Here's how the part is built. I have some questions about the finished solid (model axes, mm). Face numbers are marked on the shaded views. Coordinates: 2 decimals unless noted, no trailing zeros. Order: outer loops, then holes, each group sorted by start corner. A loop starts at its lowest first (then second) coordinate and runs counter-clockwise, first axis right, second up. Notation, with made-up numbers: (6, 24) - (63, 24) arc R28 cw to (63, 42) - close; hole circle Ø10 at (46.5, 20). An arc over 180 degrees is marked (long way). Use one line per item in the form item = value. Start each with the question number.
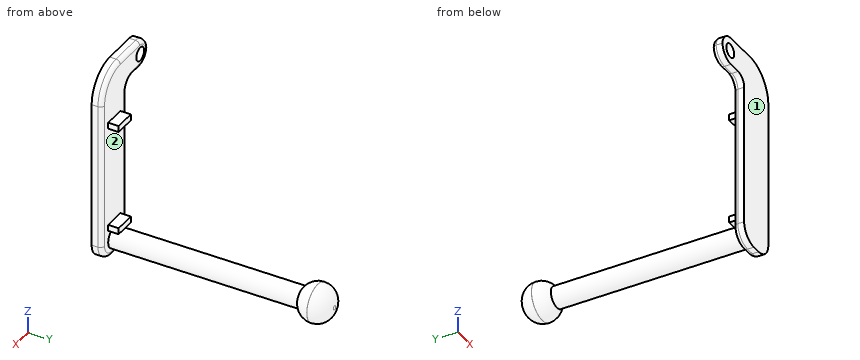
from build123d import *

# Parameters (mm, degrees)
SKETCH2_W           = 13
SKETCH2_H           = 13
SKETCH2_R           = 3.25
BOSS_EXTRUDE2_DEPTH = 5
FILLET1_R           = 15
FILLET2_R           = 5
FILLET3_R           = 7
FILLET4_R           = 2
FILLET5_R           = 8
SKETCH4_R           = 5
BOSS_EXTRUDE4_DEPTH = 90
SKETCH5_R           = 9
BOSS_EXTRUDE5_DEPTH = 15
FILLET6_R           = 8
SKETCH6_W           = 10
SKETCH6_H           = 1.5
BOSS_EXTRUDE6_DEPTH = 5
SKETCH7_W           = 10
SKETCH7_H           = 3
BOSS_EXTRUDE7_DEPTH = 5


with BuildPart() as part:
    # Sketch2 → Boss-Extrude2 (new body)
    # profile 1 of 2: a face of its own
    with BuildSketch(Plane(origin=(0, 0, 0), x_dir=(1, 0, 0), z_dir=(0, 1, 0))):
        with Locations((6.5, 6.5)):
            Rectangle(SKETCH2_W, SKETCH2_H)
        with Locations(Location((6.5, 6.5, 0), (0, 0, 270))):
            Circle(SKETCH2_R, mode=Mode.SUBTRACT)
    # profile 2 of 2: a face of its own
    with BuildSketch(Plane(origin=(0, 0, 0), x_dir=(1, 0, 0), z_dir=(0, 1, 0))):
        Polygon((13, 13), (13, 0), (38, 0), (38, 93), (18, 93), (18, 13), align=None)
    extrude(amount=BOSS_EXTRUDE2_DEPTH)

    # Fillet1
    fillet1_edges = [part.edges().sort_by_distance(p)[0] for p in [
        (38, 2.5, 0),
    ]]
    fillet(fillet1_edges, radius=FILLET1_R)

    # Fillet2
    fillet2_edges = [part.edges().sort_by_distance(p)[0] for p in [
        (18, 2.5, -13),
    ]]
    fillet(fillet2_edges, radius=FILLET2_R)

    # Fillet3
    # the kernel refuses this fillet: 7 mm, written as the material it takes off along each edge
    with BuildSketch(Plane(origin=(0, -17.5, 0), x_dir=(0, 0, -1), z_dir=(0, 1, 0)), Plane(origin=(0, -17.5, -13), x_dir=(1, 0, 0), z_dir=(0, 1, 0))) as fillet3_piece_1:
        with BuildLine():
            CenterArc((FILLET3_R, -FILLET3_R), FILLET3_R, 90, 90)
            Line((0, -FILLET3_R), (0, 0))
            Line((0, 0), (FILLET3_R, 0))
        make_face()
    extrude(amount=40, mode=Mode.SUBTRACT)

    # Fillet4
    # the kernel refuses this fillet: 2 mm, written as the material it takes off along each edge
    with BuildSketch(Plane(origin=(43, 5, -93), x_dir=(0, 0, 1), z_dir=(-1, 0, 0))) as fillet4_piece_1:
        with BuildLine():
            CenterArc((FILLET4_R, -FILLET4_R), FILLET4_R, 90, 90)
            Line((0, -FILLET4_R), (0, 0))
            Line((0, 0), (FILLET4_R, 0))
        make_face()
    extrude(amount=30, mode=Mode.SUBTRACT)
    with BuildSketch(Plane(origin=(18, 5, -98), x_dir=(1, 0, 0), z_dir=(0, 0, 1))) as fillet4_piece_2:
        with BuildLine():
            CenterArc((FILLET4_R, -FILLET4_R), FILLET4_R, 90, 90)
            Line((0, -FILLET4_R), (0, 0))
            Line((0, 0), (FILLET4_R, 0))
        make_face()
    extrude(amount=80, mode=Mode.SUBTRACT)
    with BuildSketch(Plane(origin=(38, 5, -15), x_dir=(-1, 0, 0), z_dir=(0, 0, -1))) as fillet4_piece_3:
        with BuildLine():
            CenterArc((FILLET4_R, -FILLET4_R), FILLET4_R, 90, 90)
            Line((0, -FILLET4_R), (0, 0))
            Line((0, 0), (FILLET4_R, 0))
        make_face()
    extrude(amount=83, mode=Mode.SUBTRACT)
    with BuildSketch(Plane(origin=(23, 5, -15), x_dir=(1, 0, 0), z_dir=(0, 0, -1))) as fillet4_piece_4:
        with BuildLine():
            CenterArc((15 - FILLET4_R, FILLET4_R), FILLET4_R, 270, 90)
            Line((15, FILLET4_R), (15, 0))
            Line((15, 0), (15 - FILLET4_R, 0))
        make_face()
    revolve(axis=Axis((23, 5, -15), (0, -1, 0)), revolution_arc=90, mode=Mode.SUBTRACT)
    with BuildSketch(Plane(origin=(13, 5, -18), x_dir=(0, 0, 1), z_dir=(-1, 0, 0))) as fillet4_piece_5:
        with BuildLine():
            CenterArc((5 + FILLET4_R, -FILLET4_R), FILLET4_R, 90, 90)
            Line((5, -FILLET4_R), (5, 0))
            Line((5, 0), (5 + FILLET4_R, 0))
        make_face()
    revolve(axis=Axis((13, 5, -18), (0, 1, 0)), revolution_arc=90, mode=Mode.SUBTRACT)
    with BuildSketch(Plane(origin=(23, 5, 0), x_dir=(0, 0, -1), z_dir=(-1, 0, 0))) as fillet4_piece_6:
        with BuildLine():
            CenterArc((FILLET4_R, FILLET4_R), FILLET4_R, 180, 90)
            Line((0, FILLET4_R), (0, 0))
            Line((0, 0), (FILLET4_R, 0))
        make_face()
    extrude(amount=16, mode=Mode.SUBTRACT)
    with BuildSketch(Plane(origin=(7, 5, -13), x_dir=(0, 0, 1), z_dir=(1, 0, 0))) as fillet4_piece_7:
        with BuildLine():
            CenterArc((FILLET4_R, FILLET4_R), FILLET4_R, 180, 90)
            Line((0, FILLET4_R), (0, 0))
            Line((0, 0), (FILLET4_R, 0))
        make_face()
    extrude(amount=6, mode=Mode.SUBTRACT)
    with BuildSketch(Plane(origin=(7, 5, -6), x_dir=(-0.8002659852705738, 0, 0.5996451891067899), z_dir=(0.5996451891067899, 0, 0.8002659852705738))) as fillet4_piece_8:
        with BuildLine():
            CenterArc((7 - FILLET4_R, FILLET4_R), FILLET4_R, 270, 90)
            Line((7, FILLET4_R), (7, 0))
            Line((7, 0), (7 - FILLET4_R, 0))
        make_face()
    revolve(axis=Axis((7, 5, -6), (0, -1, 0)), revolution_arc=126.844490412, mode=Mode.SUBTRACT)
    with BuildSketch(Plane(origin=(7, 5, -7), x_dir=(0, 0, 1), z_dir=(1, 0, 0))) as fillet4_piece_9:
        with BuildLine():
            CenterArc((7 - FILLET4_R, FILLET4_R), FILLET4_R, 270, 90)
            Line((7, FILLET4_R), (7, 0))
            Line((7, 0), (7 - FILLET4_R, 0))
        make_face()
    revolve(axis=Axis((7, 5, -7), (0, -1, 0)), revolution_arc=126.844490412, mode=Mode.SUBTRACT)

    # Fillet5
    # the kernel refuses this fillet: 8 mm, written as the material it takes off along each edge
    with BuildSketch(Plane(origin=(26, 5, -85), x_dir=(0, 0, -1), z_dir=(1, 0, 0))) as fillet5_piece_1:
        with BuildLine():
            CenterArc((6, -2), 2, 0, 90)
            Line((8, -2), (8, 0))
            Line((8, 0), (6, 0))
        make_face()
    revolve(axis=Axis((26, 5, -85), (0, 1, 0)), revolution_arc=90, mode=Mode.SUBTRACT)
    with BuildSketch(Plane(origin=(30, 5, -85), x_dir=(1, 0, 0), z_dir=(0, 0, 1))) as fillet5_piece_2:
        with BuildLine():
            CenterArc((6, -2), 2, 0, 90)
            Line((8, -2), (8, 0))
            Line((8, 0), (6, 0))
        make_face()
    revolve(axis=Axis((30, 5, -85), (0, 1, 0)), revolution_arc=90, mode=Mode.SUBTRACT)
    with BuildSketch(Plane(origin=(38, -20, -93), x_dir=(-1, 0, 0), z_dir=(0, 1, 0)), Plane(origin=(18, -20, -93), x_dir=(0, 0, 1), z_dir=(0, 1, 0))) as fillet5_piece_3:
        with BuildLine():
            CenterArc((FILLET5_R, FILLET5_R), FILLET5_R, 180, 90)
            Line((0, FILLET5_R), (0, 0))
            Line((0, 0), (FILLET5_R, 0))
        make_face()
    extrude(amount=25, mode=Mode.SUBTRACT)

    # Sketch4 → Boss-Extrude4 (add)
    with BuildSketch(Plane(origin=(0, 5, 0), x_dir=(1, 0, 0), z_dir=(0, 1, 0))):
        with Locations(Location((28, 85, 0), (0, 0, 90))):
            Circle(SKETCH4_R)
    extrude(amount=BOSS_EXTRUDE4_DEPTH)

    # Sketch5 → Boss-Extrude5 (add)
    with BuildSketch(Plane(origin=(0, 95, 0), x_dir=(1, 0, 0), z_dir=(0, 1, 0))):
        with Locations(Location((28, 85, 0), (0, 0, 270))):
            Circle(SKETCH5_R)
    extrude(amount=BOSS_EXTRUDE5_DEPTH)

    # Fillet6
    # the kernel refuses this fillet: 8 mm, written as the material it takes off along each edge
    with BuildSketch(Plane(origin=(28, 95, -85), x_dir=(0, 0, 1), z_dir=(-1, 0, 0))) as fillet6_piece_1:
        with BuildLine():
            CenterArc((1, 6.92820323), FILLET6_R, 300, 60)
            Line((5, 0), (5.08, -0.138564065))
            ThreePointArc((5.08, -0.138564065), (7, -0.16), (9, -0.16))
            Line((9, -0.16), (9.16, 0))
            Line((9.16, 0), (9.16, 6.92820323))
            Line((9.16, 6.92820323), (9, 6.92820323))
        make_face()
    revolve(axis=Axis((28, 95, -85), (0, 1, 0)), mode=Mode.SUBTRACT)
    with BuildSketch(Plane(origin=(28, 110, -85), x_dir=(0, 0, 1), z_dir=(-1, 0, 0))) as fillet6_piece_2:
        with BuildLine():
            CenterArc((9 - FILLET6_R, -FILLET6_R), FILLET6_R, 0, 90)
            Line((9 - FILLET6_R, 0), (9 - FILLET6_R, FILLET6_R * 0.02))
            Line((9 - FILLET6_R, FILLET6_R * 0.02), (9 + FILLET6_R * 0.02, FILLET6_R * 0.02))
            Line((9 + FILLET6_R * 0.02, FILLET6_R * 0.02), (9 + FILLET6_R * 0.02, -FILLET6_R))
            Line((9 + FILLET6_R * 0.02, -FILLET6_R), (9, -FILLET6_R))
        make_face()
    revolve(axis=Axis((28, 110, -85), (0, 1, 0)), mode=Mode.SUBTRACT)

    # Sketch6 → Boss-Extrude6 (add)
    with BuildSketch(Plane(origin=(0, 5, 0), x_dir=(1, 0, 0), z_dir=(0, 1, 0))):
        with Locations((28, 25.944405325)):
            Rectangle(SKETCH6_W, SKETCH6_H)
        with Locations((28, 27.444405325)):
            Rectangle(SKETCH6_W, SKETCH6_H)
    extrude(amount=BOSS_EXTRUDE6_DEPTH)

    # Sketch7 → Boss-Extrude7 (add)
    with BuildSketch(Plane(origin=(0, 5, 0), x_dir=(1, 0, 0), z_dir=(0, 1, 0))):
        with Locations((28, 77.6172361)):
            Rectangle(SKETCH7_W, SKETCH7_H)
    extrude(amount=BOSS_EXTRUDE7_DEPTH)


solid = part.part
1) Suppose I cut it at A-A, the plane z = -59. List the corners of the cut face in (x, y) for me.
2) If we mould it in two halves opening along Z, with no side actions, what happens to the marked faces 1 and 2? For each: pulls with the +Z half, pulls with the -Z half, needs draft (parallel to the pull), parting line crosses it, or undercut.
3) Suppose I cut it at B-B, the plane y = 62. List the corners of the cut face in (x, z) for me, then the cut area to 3 significant figures.
4) I need wall thicknesses on probe 1 along Z at (x, y) = (28, 64); probe 2 along Y at (x, z) = (29, -63); probe 3 along X at (y, z) = (3, -6). Which ranges of each line are inside material? Lowest first, please. Write a range as [from, to].
5) For pin 1 (4 mm diameter, centred on x = 29, y = 8.5, fed in from +Z); pin 2 (3.5 mm diameter, centred on x = 29, y = 1, fed in from -Z); pin 3 (3.5 mm diameter, centred on y = 7.5, z = -77.5, fed in from -X), each with a flat end and sliding along its axis, tell me the tip position at first contact or that it passes through.
From the geometry:
q1.outline = (18, 0) - (38, 0) - (38, 3) arc R2 ccw to (36, 5) - (20, 5) arc R2 ccw to (18, 3) - close
q2.face_1 = needs draft
q2.face_2 = undercut
q3.outline = circle Ø10 at (28, -85)
q3.area = 78.5 mm2
q4.probe_1 = [-90, -80]
q4.probe_2 = [0, 5]
q4.probe_3 = [0.07, 3.29], [9.71, 35]
q5.pin_1 = -25.19
q5.pin_2 = -93
q5.pin_3 = 23
